from build123d import *

# Parameters (mm, degrees)
SKETCH064_W     = 445
SKETCH064_H     = 232
PAD024_DEPTH    = 3
SKETCH065_R     = 9.5
POCKET040_DEPTH = 5
FILLET009_R     = 2
SKETCH066_R     = 7
POCKET041_DEPTH = 10.001
SKETCH081_W     = 425.970062
SKETCH081_H     = 417.705674
POCKET053_DEPTH = 5


with BuildPart() as part:
    # Sketch064 → Pad024 (new body)
    with BuildSketch(Plane.XY):
        Rectangle(SKETCH064_W, SKETCH064_H)
    extrude(amount=PAD024_DEPTH)

    # Sketch065 (on Face6 of Pad024) → Pocket040 (cut)
    with BuildSketch(Plane.XY.offset(3)):
        with Locations((-171, 55)):
            Circle(SKETCH065_R)
        with Locations((-171, 33)):
            Circle(SKETCH065_R)
        with Locations((-171, 11)):
            Circle(SKETCH065_R)
        with Locations((-171, -11)):
            Circle(SKETCH065_R)
        with Locations((-171, -33)):
            Circle(SKETCH065_R)
        with Locations((-171, -55)):
            Circle(SKETCH065_R)
        with Locations((-152, 44)):
            Circle(SKETCH065_R)
        with Locations((-152, 22)):
            Circle(SKETCH065_R)
        with Locations((-152, 0)):
            Circle(SKETCH065_R)
        with Locations((-152, -22)):
            Circle(SKETCH065_R)
        with Locations((-152, -44)):
            Circle(SKETCH065_R)
        with Locations((-133, 55)):
            Circle(SKETCH065_R)
        with Locations((-133, 33)):
            Circle(SKETCH065_R)
        with Locations((-133, 11)):
            Circle(SKETCH065_R)
        with Locations((-133, -11)):
            Circle(SKETCH065_R)
        with Locations((-133, -33)):
            Circle(SKETCH065_R)
        with Locations((-133, -55)):
            Circle(SKETCH065_R)
        with Locations((-114, 44)):
            Circle(SKETCH065_R)
        with Locations((-114, 22)):
            Circle(SKETCH065_R)
        with Locations((-114, 0)):
            Circle(SKETCH065_R)
        with Locations((-114, -22)):
            Circle(SKETCH065_R)
        with Locations((-114, -44)):
            Circle(SKETCH065_R)
        with Locations((-95, 55)):
            Circle(SKETCH065_R)
        with Locations((-95, 33)):
            Circle(SKETCH065_R)
        with Locations((-95, 11)):
            Circle(SKETCH065_R)
        with Locations((-95, -11)):
            Circle(SKETCH065_R)
        with Locations((-95, -33)):
            Circle(SKETCH065_R)
        with Locations((-95, -55)):
            Circle(SKETCH065_R)
        with Locations((-76, -44)):
            Circle(SKETCH065_R)
        with Locations((-76, -22)):
            Circle(SKETCH065_R)
        with Locations((-76, 0)):
            Circle(SKETCH065_R)
        with Locations((-76, 22)):
            Circle(SKETCH065_R)
        with Locations((-76, 44)):
            Circle(SKETCH065_R)
        with Locations((-57, 55)):
            Circle(SKETCH065_R)
        with Locations((-57, 33)):
            Circle(SKETCH065_R)
        with Locations((-57, 11)):
            Circle(SKETCH065_R)
        with Locations((-57, -11)):
            Circle(SKETCH065_R)
        with Locations((-57, -33)):
            Circle(SKETCH065_R)
        with Locations((-38, 44)):
            Circle(SKETCH065_R)
        with Locations((-38, 22)):
            Circle(SKETCH065_R)
        with Locations((-38, 0)):
            Circle(SKETCH065_R)
        with Locations((-38, -22)):
            Circle(SKETCH065_R)
        with Locations((-38, -44)):
            Circle(SKETCH065_R)
        with Locations((-57, -55)):
            Circle(SKETCH065_R)
        with Locations((-19, 55)):
            Circle(SKETCH065_R)
        with Locations((-19, 33)):
            Circle(SKETCH065_R)
        with Locations((-19, 11)):
            Circle(SKETCH065_R)
        with Locations((-19, -11)):
            Circle(SKETCH065_R)
        with Locations((-19, -33)):
            Circle(SKETCH065_R)
        with Locations((-19, -55)):
            Circle(SKETCH065_R)
        with Locations((0, -44)):
            Circle(SKETCH065_R)
        with Locations((0, -22)):
            Circle(SKETCH065_R)
        Circle(SKETCH065_R)
        with Locations((0, 22)):
            Circle(SKETCH065_R)
        with Locations((0, 44)):
            Circle(SKETCH065_R)
        with Locations((19, 55)):
            Circle(SKETCH065_R)
        with Locations((19, 33)):
            Circle(SKETCH065_R)
        with Locations((19, 11)):
            Circle(SKETCH065_R)
        with Locations((19, -11)):
            Circle(SKETCH065_R)
        with Locations((19, -33)):
            Circle(SKETCH065_R)
        with Locations((19, -55)):
            Circle(SKETCH065_R)
        with Locations((38, -44)):
            Circle(SKETCH065_R)
        with Locations((38, -22)):
            Circle(SKETCH065_R)
        with Locations((38, 0)):
            Circle(SKETCH065_R)
        with Locations((38, 22)):
            Circle(SKETCH065_R)
        with Locations((38, 44)):
            Circle(SKETCH065_R)
        with Locations((57, 55)):
            Circle(SKETCH065_R)
        with Locations((57, 33)):
            Circle(SKETCH065_R)
        with Locations((57, 11)):
            Circle(SKETCH065_R)
        with Locations((57, -11)):
            Circle(SKETCH065_R)
        with Locations((76, 0)):
            Circle(SKETCH065_R)
        with Locations((76, 22)):
            Circle(SKETCH065_R)
        with Locations((76, 44)):
            Circle(SKETCH065_R)
        with Locations((57, -33)):
            Circle(SKETCH065_R)
        with Locations((57, -55)):
            Circle(SKETCH065_R)
        with Locations((76, -44)):
            Circle(SKETCH065_R)
        with Locations((76, -22)):
            Circle(SKETCH065_R)
        with Locations((95, 55)):
            Circle(SKETCH065_R)
        with Locations((95, 33)):
            Circle(SKETCH065_R)
        with Locations((95, 11)):
            Circle(SKETCH065_R)
        with Locations((95, -11)):
            Circle(SKETCH065_R)
        with Locations((95, -33)):
            Circle(SKETCH065_R)
        with Locations((95, -55)):
            Circle(SKETCH065_R)
        with Locations((114, 44)):
            Circle(SKETCH065_R)
        with Locations((114, 22)):
            Circle(SKETCH065_R)
        with Locations((114, 0)):
            Circle(SKETCH065_R)
        with Locations((114, -22)):
            Circle(SKETCH065_R)
        with Locations((114, -44)):
            Circle(SKETCH065_R)
        with Locations((133, 55)):
            Circle(SKETCH065_R)
        with Locations((133, 33)):
            Circle(SKETCH065_R)
        with Locations((133, 11)):
            Circle(SKETCH065_R)
        with Locations((133, -11)):
            Circle(SKETCH065_R)
        with Locations((133, -33)):
            Circle(SKETCH065_R)
        with Locations((133, -55)):
            Circle(SKETCH065_R)
        with Locations((152, 44)):
            Circle(SKETCH065_R)
        with Locations((152, 22)):
            Circle(SKETCH065_R)
        with Locations((152, 0)):
            Circle(SKETCH065_R)
        with Locations((152, -22)):
            Circle(SKETCH065_R)
        with Locations((152, -44)):
            Circle(SKETCH065_R)
        with Locations((171, 55)):
            Circle(SKETCH065_R)
        with Locations((171, 33)):
            Circle(SKETCH065_R)
        with Locations((171, 11)):
            Circle(SKETCH065_R)
        with Locations((171, -11)):
            Circle(SKETCH065_R)
        with Locations((171, -33)):
            Circle(SKETCH065_R)
        with Locations((171, -55)):
            Circle(SKETCH065_R)
    extrude(amount=-POCKET040_DEPTH, mode=Mode.SUBTRACT)

    # Fillet009
    fillet009_edges = [part.edges().sort_by_distance(p)[0] for p in [
        (-222.5, -116, 1.5),
        (222.5, -116, 1.5),
        (222.5, 116, 1.5),
        (-222.5, 116, 1.5),
    ]]
    fillet(fillet009_edges, radius=FILLET009_R)

    # Sketch066 → Pocket041 (cut, through all)
    with BuildSketch(Plane.XY.offset(10)):
        with Locations((197.939534, 0)):
            Circle(SKETCH066_R)
    extrude(amount=-POCKET041_DEPTH, mode=Mode.SUBTRACT)

    # Sketch081 (on Face5 of Pocket041) → Pocket053 (cut)
    with BuildSketch(Plane.XY.offset(3)):
        with Locations((117.985031, -23.346199)):
            Rectangle(SKETCH081_W, SKETCH081_H)
    extrude(amount=-POCKET053_DEPTH, mode=Mode.SUBTRACT)


solid = part.part
The listing builds one solid part. Answer for the finished solid, in the listing's coordinates (mm). Give positions to 0.01 mm unless a question says otherwise; leave off trailing zeros. Write each loop counter-clockwise with the first axis right and the second up, starting at its lowest first coordinate (ties: lowest second). Pieces come first, ordered by that corner, then holes. Notation, with made-up numbers: (11.5, -22.5) - (36.5, -22.5) arc R25 ccw to (36.5, -10.5) - close; hole circle Ø11 at (-18, -28.75). An arc over 180 degrees is marked (long way). Use a Markdown table: item, result.
1. For a pull along X with two mould halves and no side action, classify faces 1 (the cylindrical face through (-140, 39.42, 1.52)), 2 (the flat face through (-173.8, 1.6, 0)), 3 (the cylindrical face through (-104.498, 33.209, 1.521)), 4 (the cylindrical face through (-142.49, -10.58, 1.52)) as released by +X, released by -X, zero draft, split by the parting line, or undercut.
Values follow:
| item | result |
|---|---|
| face 1 | undercut |
| face 2 | zero draft |
| face 3 | released by +X |
| face 4 | undercut |
2. Find the intervals of material crossed by probe 1 along Y at (x, z) = (-114, 1.4); probe 2 along X at (y, z) = (-21.5, 2.8); probe 3 along Y at (x, z) = (-116.5, 1.2), in increasing order. Write a range as from..to.
Values follow:
| item | result |
|---|---|
| probe 1 | y = -116..-53.5, -34.5..-31.5, -12.5..-9.5, 9.5..12.5, 31.5..34.5, 53.5..116 |
| probe 2 | x = -222.5..-161.49, -142.51..-123.49, -104.51..-95 |
| probe 3 | y = -116..-53.17, -34.83..-31.17, -12.83..-9.17, 9.17..12.83, 31.17..34.83, 53.17..116 |
3. Section C-C on z = 1.2 is taken. Count the separate pieces of the cut face and the enclosed holes in it, plus the area to 3 significant figures.
Values follow:
| item | result |
|---|---|
| separate pieces | 1 |
| enclosed holes | 22 |
| area | 22,500 mm² |
4. Section A-A on x = -114 is taken. Write down the section's boundary in (y, z), plus the area to 3 significant figures.
Values follow:
| item | result |
|---|---|
| outline | (-116, 0) - (-53.5, 0) - (-53.5, 3) - (-116, 3) - close; (-34.5, 0) - (-31.5, 0) - (-31.5, 3) - (-34.5, 3) - close; (-12.5, 0) - (-9.5, 0) - (-9.5, 3) - (-12.5, 3) - close; (9.5, 0) - (12.5, 0) - (12.5, 3) - (9.5, 3) - close; (31.5, 0) - (34.5, 0) - (34.5, 3) - (31.5, 3) - close; (53.5, 0) - (116, 0) - (116, 3) - (53.5, 3) - close |
| area | 411 mm² |
5. Section B-B on x = -171 is taken. Write down the section's boundary in (y, z), plus the area to 3 significant figures.
Values follow:
| item | result |
|---|---|
| outline | (-116, 0) - (-64.5, 0) - (-64.5, 3) - (-116, 3) - close; (-45.5, 0) - (-42.5, 0) - (-42.5, 3) - (-45.5, 3) - close; (-23.5, 0) - (-20.5, 0) - (-20.5, 3) - (-23.5, 3) - close; (-1.5, 0) - (1.5, 0) - (1.5, 3) - (-1.5, 3) - close; (20.5, 0) - (23.5, 0) - (23.5, 3) - (20.5, 3) - close; (42.5, 0) - (45.5, 0) - (45.5, 3) - (42.5, 3) - close; (64.5, 0) - (116, 0) - (116, 3) - (64.5, 3) - close |
| area | 354 mm² |
